from build123d import *

# Parameters (mm, degrees)
F1_DEPTH = 97.5
F2_R     = 3.1
F3_DEPTH = 25
F4_R     = 2.5
F5_R     = 1


with BuildPart() as f1:
    # F0 (on Front) → F1 (new body, symmetric)
    with BuildSketch(Plane.XZ):
        Polygon((0, 30), (0, 0), (1.5, 0), (1.5, 28.5), (58, 28.5), (58, 30), align=None)
    extrude(amount=F1_DEPTH, both=True)

    # F2 (on face) → F3 (cut)
    with BuildSketch(Plane(origin=(0, 0, 0), x_dir=(0, -1, 0), z_dir=(-1, 0, 0))):
        with Locations((-85.6, 10)):
            Circle(F2_R)
        with Locations((85.6, 10)):
            Circle(F2_R)
    extrude(amount=-F3_DEPTH, mode=Mode.SUBTRACT)

    # F4
    f4_edges = [f1.edges().sort_by_distance(p)[0] for p in [
        (0, 0, 30),
    ]]
    fillet(f4_edges, radius=F4_R)

    # F5
    f5_edges = [f1.edges().sort_by_distance(p)[0] for p in [
        (1.5, 0, 28.5),
    ]]
    fillet(f5_edges, radius=F5_R)


solid = f1.part
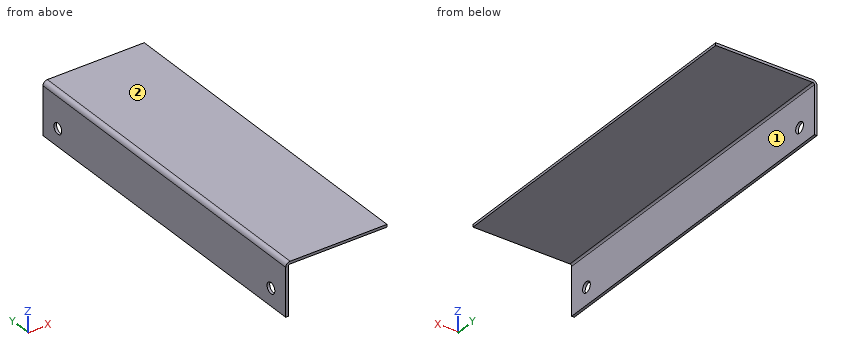
Geometry check sheet. Reference: the model listing, model coordinates, mm. Face numbers are marked on the shaded views. A direction names the side the tool comes from. Coordinates: 2 decimals unless noted, no trailing zeros. Order: outer loops, then holes, each group sorted by start corner. A loop starts at its lowest first (then second) coordinate and runs counter-clockwise, first axis right, second up. Notation, with made-up numbers: M 17,-38.75 L 67,-38.75 A24 cw 67,-2.75 Z; hole C -32.75,32.5 d1. An arc over 180 degrees is marked long. Use CSV: the item, a comma, the result in double quotes.
Item 1: Cross-section at C-C on y = 23. Record the cut outline in (x, z).
Returned:
outline,"M 0,0 L 1.5,0 L 1.5,27.5 A1 cw 2.5,28.5 L 58,28.5 L 58,30 L 2.5,30 A2.5 ccw 0,27.5 Z"
Item 2: Tool access check on the marked faces 1 and 2. Record the directions out of +Z, -Z, +X, -X, +Y, -Y that give a thin tool (end or side, any length) a straight path to the whole face; none if there is none.
Returned:
face 1,"-Z, +X, +Y, -Y"
face 2,"+Z, +X, -X, +Y, -Y"
Item 3: Cross-section at D-D on z = 21.75. Record the cut outline in (x, y), then the cut area to 4 significant figures.
Returned:
outline,"M 0,-97.5 L 1.5,-97.5 L 1.5,97.5 L 0,97.5 Z"
area,"292.5 mm2"
Item 4: Gauge pin test, flat ends, axial feed: pin 1 Ø14 at (y, z) = (27, 18.5) entering from +X; pin 2 Ø8 at (x, y) = (28, -11) entering from -Z. Record the tip position at first contact, or that the pin passes through.
Returned:
pin 1,"stops at x = 1.5"
pin 2,"stops at z = 28.5"
Item 5: Cross-section at A-A on y = -85.6. Record the cut outline in (x, z).
Returned:
outline,"M 0,0 L 1.5,0 L 1.5,6.9 L 0,6.9 Z; M 0,13.1 L 1.5,13.1 L 1.5,27.5 A1 cw 2.5,28.5 L 58,28.5 L 58,30 L 2.5,30 A2.5 ccw 0,27.5 Z"
Item 6: Thickness scan on line 1 along X through (y, z) = (-5.5, 5); line 2 along Z through (x, y) = (49, 40); line 3 along Z through (x, y) = (1.1, 85.6). Record the ranges inside material, lowest first.
Returned:
line 1,"x = 0 to 1.5"
line 2,"z = 28.5 to 30"
line 3,"z = 0 to 6.9, 13.1 to 29.57"
Item 7: Cross-section at B-B on z = 10. Record the cut outline in (x, y).
Returned:
outline,"M 0,-97.5 L 1.5,-97.5 L 1.5,-88.7 L 0,-88.7 Z; M 0,-82.5 L 1.5,-82.5 L 1.5,82.5 L 0,82.5 Z; M 0,88.7 L 1.5,88.7 L 1.5,97.5 L 0,97.5 Z"
